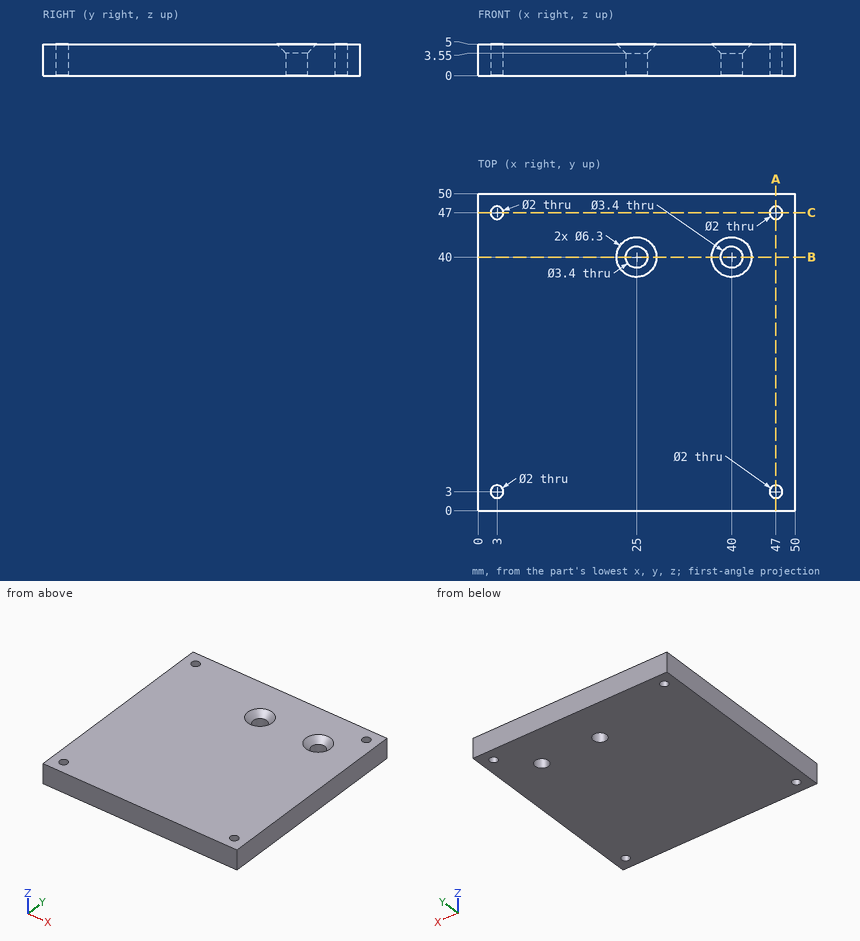
Geometry: see drawing. Coordinates: mm, zero at the bounding-box minimum. Give positions to 0.01 mm unless a question says otherwise; leave off trailing zeros. Loops run counter-clockwise (first coordinate to the right, second up) from the corner with the lowest first, then second, coordinate; pieces in that order, holes last. Notation, with made-up numbers: (87.5, 27.25) - (105.5, 27.25) arc R11 ccw to (105.5, 34.25) - close; hole circle Ø11 at (-38, -8). An arc over 180 degrees is marked (long way). Use CSV: the item, a comma, the result in double quotes. Start each with the question number.
1. Ray query, L1, parallel to Y at x = 47, z = 1.65; L2, parallel to Y at x = 40, z = 2.75; L3, parallel to X at y = 41, z = 3.1. Return the intervals inside material, ascending.
2. Section B-B (y = 40). Output: boundary loops of the cut face in (x, z), then the cut area to 3 significant figures.
3. Section A-A (x = 47). Output: boundary loops of the cut face in (y, z), then the cut area to 3 significant figures.
4. Pin query (flat end, axial travel): pin 1 (3 mm diameter, centred on x = 47, y = 47, fed in from +Z); pin 2 (4 mm diameter, centred on x = 25, y = 40, fed in from +Z). Return the tip coordinate at first contact, or that it passes through.
Response:
1,L1,"0 to 2, 4 to 46, 48 to 50"
1,L2,"0 to 38.3, 41.7 to 50"
1,L3,"0 to 23.63, 26.37 to 38.63, 41.37 to 50"
2,outline,"(0, 0) - (23.3, 0) - (23.3, 3.55) - (21.85, 5) - (0, 5) - close; (26.7, 0) - (38.3, 0) - (38.3, 3.55) - (36.85, 5) - (28.15, 5) - (26.7, 3.55) - close; (41.7, 0) - (50, 0) - (50, 5) - (43.15, 5) - (41.7, 3.55) - close"
2,area,"212 mm²"
3,outline,"(0, 0) - (2, 0) - (2, 5) - (0, 5) - close; (4, 0) - (46, 0) - (46, 5) - (4, 5) - close; (48, 0) - (50, 0) - (50, 5) - (48, 5) - close"
3,area,"230 mm²"
4,pin 1,"z = 5"
4,pin 2,"z = 3.85"
